The model under review builds one solid part; all positions refer to its coordinate system, in mm. Face numbers are marked on the shaded views. A direction names the side the tool comes from. Coordinates: 2 decimals unless noted, no trailing zeros. Order: outer loops, then holes, each group sorted by start corner. A loop starts at its lowest first (then second) coordinate and runs counter-clockwise, first axis right, second up. Notation, with made-up numbers: M 26.25,82 L 42.25,82 A16 ccw 42.25,89 Z; hole C -31,66 d9. An arc over 180 degrees is marked long. Write each question's results on one line, items separated by ' | '.
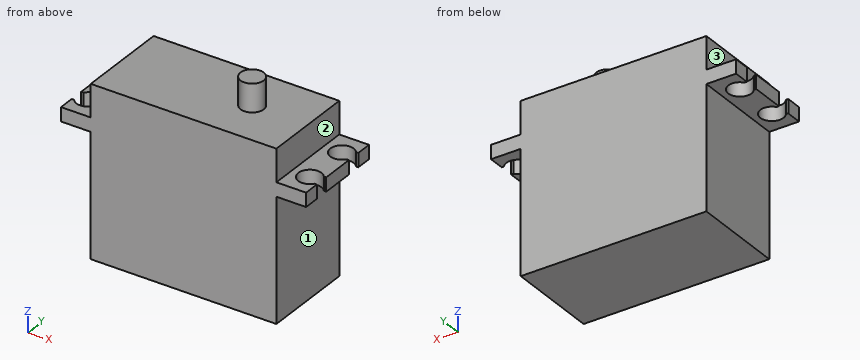
Autodesk Inventor part; units mm, degrees
ref_plane "YZ Plane" through (0, 0, 0) normal (1, 0, 0) x (0, 1, 0)
ref_plane "XZ Plane" through (0, 0, 0) normal (0, 1, 0) x (-1, 0, 0)
ref_plane "XY Plane" through (0, 0, 0) normal (0, 0, 1) x (1, 0, 0)
sketch "草圖1" plane through (0, 0, 0) normal (0, 1, 0) x (-1, 0, 0)
  line L0 (20, -18.25) -> (-20, -18.25)
  line L1 (-20, -18.25) -> (-20, 18.25)
  line L2 (-20, 18.25) -> (20, 18.25)
  line L3 (20, 18.25) -> (20, -18.25)
  line L4 (20, -18.25) -> (-20, 18.25) construction
  line L5 (-20, -18.25) -> (20, 18.25) construction
  line L6 (26.4, 11.25) -> (-26.4, 11.25)
  line L7 (-26.4, 11.25) -> (-26.4, 8.25)
  line L8 (-26.4, 8.25) -> (26.4, 8.25)
  line L9 (26.4, 8.25) -> (26.4, 11.25)
  point P0 (0, 0)
  point P1 (0, 11.25)
  point P2 (0, 18.25)
  dimension "d0" = 40
  dimension "d1" = 36.5
  dimension "d2" = 3
  dimension "d4" = 52.8
  dimension "d5" = 26.5
extrude "擠出1" add sketch "草圖1" along normal mid plane 20
sketch "草圖2" plane through (20, -10, 11.25) normal (0, 0, 1) x (1, 0, 0)
  line L0 (-40, 0) -> (-40, 20) construction
  line L1 (0, 20) -> (-40, 20) construction
  line L2 (0, 20) -> (0, 0) construction
  line L3 (-40, 0) -> (0, 0) construction
  line L4 (-43.9, 4.9) -> (3.9, 4.9) construction
  line L5 (3.9, 4.9) -> (3.9, 15.1) construction
  line L6 (3.9, 15.1) -> (-43.9, 15.1) construction
  line L7 (-43.9, 15.1) -> (-43.9, 4.9) construction
  line L8 (-43.9, 4.9) -> (3.9, 15.1) construction
  line L9 (3.9, 4.9) -> (-43.9, 15.1) construction
  point P0 (-20, 10)
  dimension "d8" = 47.8
  dimension "d9" = 10.2
hole "孔1" at (23.9, 5.1, 11.25) at (23.9, -5.1, 11.25) at (-23.9, -5.1, 11.25) at (-23.9, 5.1, 11.25) direction (0, 0, -1) diameter 5 depth 8 tip angle 118
sketch "草圖3" plane through (20, -10, 11.25) normal (0, 0, 1) x (1, 0, 0)
  circle A0 centre (3.9, 15.1) radius 2.5 construction
  line L0 (3.9, 16.6) -> (13.7017, 16.6)
  line L1 (13.7017, 16.6) -> (13.7017, 13.6)
  line L2 (13.7017, 13.6) -> (3.9, 13.6)
  line L3 (3.9, 13.6) -> (3.9, 16.6)
  point P0 (-20, 10)
  point P1 (6.4, 15.1)
  dimension "d17" = 3
extrude "擠出2" cut sketch "草圖3" against normal blind 20
mirror "鏡射1" about plane through (0, 0, 0) normal (0, 1, 0) of "擠出2"
mirror "鏡射2" about plane through (0, 0, 0) normal (1, 0, 0) of "擠出2", "鏡射1"
sketch "草圖4" plane through (-20, 10, 18.25) normal (0, 0, 1) x (1, 0, 0)
  circle A0 centre (28, -10) radius 2.5
  line L0 (40, 0) -> (40, -20) construction
  line L1 (0, 0) -> (0, -20)
  point P0 (20, -10)
  dimension "d20" = 5
  dimension "d25" = 12
extrude "擠出3" add sketch "草圖4" along normal blind 6
properties part number "馬達"
1) Take a section at B-B on y = 5.1. State the section outline as (x, z) points, plus the area to 3 significant figures.
Solutions:
outline: M -21.4,8.25 L -20,8.25 L -20,-18.25 L 20,-18.25 L 20,8.25 L 21.4,8.25 L 21.4,11.25 L 20,11.25 L 20,18.25 L -20,18.25 L -20,11.25 L -21.4,11.25 Z | area: 1,470 mm2
2) Take a section at C-C on x = 8. State the section outline as (y, z) points, plus the area to 3 significant figures.
Solutions:
outline: M -10,-18.25 L 10,-18.25 L 10,18.25 L 2.5,18.25 L 2.5,24.25 L -2.5,24.25 L -2.5,18.25 L -10,18.25 Z | area: 760 mm2
3) Take a section at A-A on x = 23.9. State the section outline as (y, z) points.
Solutions:
outline: M -10,8.25 L -7.6,8.25 L -7.6,11.25 L -10,11.25 Z; M -2.6,8.25 L 2.6,8.25 L 2.6,11.25 L -2.6,11.25 Z; M 7.6,8.25 L 10,8.25 L 10,11.25 L 7.6,11.25 Z
4) For the marked faces 1, 2 and 3, list the 3-axis set-ups (+Z, -Z, +X, -X, +Y, -Y) from which the entire face can be reached by the end or side of a thin tool; tool diameter is ignored.
Solutions:
face 1: -Z, +X, +Y, -Y | face 2: +Z, +X, +Y, -Y | face 3: +Z, -X, +Y, -Y
5) Take a section at D-D on z = 5. State the section outline as (x, y) points, plus the area to 3 significant figures.
Solutions:
outline: M -20,-10 L 20,-10 L 20,10 L -20,10 Z | area: 800 mm2
6) To check wall thickness, follow line 1 along Y through (x, z) = (-23.9, 9.05); line 2 along Y through (x, z) = (23, 9); line 3 along X through (y, z) = (-4.5, 17). State the ranges of each line that lie inside material, in increasing order.
Solutions:
line 1: -10 to -7.6, -2.6 to 2.6, 7.6 to 10 | line 2: -10 to -7.43, -2.77 to 2.77, 7.43 to 10 | line 3: -20 to 20
7) For pin 1 (5 mm diameter, centred on x = 3.5, y = -6, fed in from +Z); pin 2 (1.5 mm diameter, centred on y = -3.5, z = 1.5, fed in from +X); pin 3 (3 mm diameter, centred on x = 22, y = -4.5, fed in from +Z), all flat-tipped, find the tip position at first contact; note any pin that passes through.
Solutions:
pin 1: z = 18.25 | pin 2: x = 20 | pin 3: z = 11.25
